Model file for the job. Use its own axes, mm. A direction names the side the tool comes from. Coordinates: 2 decimals unless noted, no trailing zeros. Order: outer loops, then holes, each group sorted by start corner. A loop starts at its lowest first (then second) coordinate and runs counter-clockwise, first axis right, second up. Notation, with made-up numbers: (26, 44.25) -> (60, 44.25) arc R27 cw to (60, 62.25) -> close; hole circle Ø9 at (82.5, 24). An arc over 180 degrees is marked (long way). Return JSON: item names as keys, results as strings. Group by question number.
1) Cut at D-D (z = -16.5). Write the cut outline in (x, y).
2) Flat gauge pins, fed straight in: pin 1 (1 mm diameter, centred on x = 3.5, y = 0.5, fed in from +Z); pin 2 (1 mm diameter, centred on y = 1.5, z = -17, fed in from -X). Where does each tip first touch, or does it go through?
3) Cut at A-A (y = 1.6). Write the cut outline in (x, z) (3 decimals), and give its area (3 significant figures).
4) Pull direction X, two halves, no side cores. Call faces 1 (the flat face through (14.42, 1.01, -18.83)), 2 (the cylindrical face through (-21.145, 1.014, -27.287)), 3 (the flat face through (0, 0, -15)): +X half, -X half, draft (parallel to the pull), parting line (faces both ways), or undercut.
5) Probe line 1 (Z direction, x = -14.5, y = 1.6); line 2 (X direction, y = 0.4, z = -23.5); line 3 (Z direction, x = -14, y = 1.7). List the from-to ranges inside material, lowest first.
6) Which spindle directions (+Z, -Z, +X, -X, +Y, -Y) get a long thin tool onto all of the face, cutting with end or side? Do faces 4 (the cylindrical face through (-19.607, 1.014, -22.597)), 5 (the cylindrical face through (10.805, 1.014, -26.908)), 6 (the flat face through (-14.387, 1.014, -18.877)), 7 (the flat face through (25.863, 1, -26)). Say none if no direction does.
7) Cut at B-B (z = -25.75). Write the cut outline in (x, y), and give its area (3 significant figures).
8) Cut at C-C (x = 0). Write the cut outline in (y, z) (3 decimals).
from build123d import *

# Parameters (mm, degrees)
BOSS_EXTRUDE1_DEPTH = 2
SKETCH5_W           = 68.030538665
SKETCH5_H           = 29.277015507
CUT_EXTRUDE3_DEPTH  = 2


with BuildPart() as part:
    # Sketch3 → Boss-Extrude1 (new body)
    with BuildSketch(Plane(origin=(0, 0, 0), x_dir=(1, 0, 0), z_dir=(0, 1, 0))):
        with BuildLine():
            Line((-13.637639272, 20.383278482), (-15.860247962, 17.20906431))
            ThreePointArc((-15.860247962, 17.20906431), (-13.666207185, 14.707240293), (-12.875283017, 11.475))
            ThreePointArc((-12.875283017, 11.475), (-10.092914311, 8.804356775), (-6.237643745, 8.908278482))
            ThreePointArc((-6.237643745, 8.908278482), (0, 10.875), (6.237643745, 8.908278482))
            ThreePointArc((6.237643745, 8.908278482), (10.092914311, 8.804356775), (12.875283017, 11.475))
            ThreePointArc((12.875283017, 11.475), (13.666207185, 14.707240293), (15.860247962, 17.20906431))
            Line((15.860247962, 17.20906431), (13.637639272, 20.383278482))
            ThreePointArc((13.637639272, 20.383278482), (19.875283017, 22.35), (26.112926762, 20.383278482))
            Line((26.112926762, 20.383278482), (26.112926762, 31.248240565))
            ThreePointArc((26.112926762, 31.248240565), (21.575193898, 27.634543241), (15.870079226, 28.68406431))
            ThreePointArc((15.870079226, 28.68406431), (10.616247764, 27.083629141), (7, 22.95))
            ThreePointArc((7, 22.95), (0, 15.95), (-7, 22.95))
            ThreePointArc((-7, 22.95), (-10.616247764, 27.083629141), (-15.870079226, 28.68406431))
            ThreePointArc((-15.870079226, 28.68406431), (-21.575193898, 27.634543241), (-26.112926762, 31.248240565))
            Line((-26.112926762, 31.248240565), (-26.112926762, 20.383278482))
            ThreePointArc((-26.112926762, 20.383278482), (-19.875283017, 22.35), (-13.637639272, 20.383278482))
        make_face()
    extrude(amount=BOSS_EXTRUDE1_DEPTH)

    # Sketch5 → Cut-Extrude3 (cut)
    with BuildSketch(Plane(origin=(0, 2, 0), x_dir=(1, 0, 0), z_dir=(0, 1, 0))):
        with Locations((1.906858247, 20.166215681)):
            Rectangle(SKETCH5_W, SKETCH5_H)
        with BuildLine():
            Line((25.862926762, 20.851233112), (25.862926762, 30.337137187))
            ThreePointArc((25.862926762, 30.337137187), (21.222970901, 27.301360666), (15.794718469, 28.432380125))
            ThreePointArc((15.794718469, 28.432380125), (10.741632002, 26.866985754), (7.249777379, 22.893184845))
            ThreePointArc((7.249777379, 22.893184845), (0, 15.7), (-7.249777379, 22.893184845))
            ThreePointArc((-7.249777379, 22.893184845), (-10.741632002, 26.866985754), (-15.794718469, 28.432380125))
            ThreePointArc((-15.794718469, 28.432380125), (-21.222970901, 27.301360666), (-25.862926762, 30.337137187))
            Line((-25.862926762, 30.337137187), (-25.862926762, 20.851233112))
            ThreePointArc((-25.862926762, 20.851233112), (-19.513666923, 22.594121314), (-13.291068525, 20.442371104))
            Line((-13.291068525, 20.442371104), (-15.51453889, 17.266926334))
            ThreePointArc((-15.51453889, 17.266926334), (-13.399579679, 14.735025503), (-12.625477511, 11.528104843))
            ThreePointArc((-12.625477511, 11.528104843), (-9.989809939, 9.032549256), (-6.361359115, 9.126814078))
            ThreePointArc((-6.361359115, 9.126814078), (0, 11.125), (6.361359115, 9.126814078))
            ThreePointArc((6.361359115, 9.126814078), (9.989809939, 9.032549256), (12.625477511, 11.528104843))
            ThreePointArc((12.625477511, 11.528104843), (13.399579679, 14.735025503), (15.51453889, 17.266926334))
            Line((15.51453889, 17.266926334), (13.291068525, 20.442371104))
            ThreePointArc((13.291068525, 20.442371104), (19.513666923, 22.594121314), (25.862926762, 20.851233112))
        make_face(mode=Mode.SUBTRACT)
    extrude(amount=-CUT_EXTRUDE3_DEPTH, mode=Mode.SUBTRACT)


solid = part.part
Answers below:
{
 "1": {"outline": "(-14.65, 0) -> (-3.31, 0) -> (-3.31, 2) -> (-14.65, 2) -> close; (3.31, 0) -> (14.65, 0) -> (14.65, 2) -> (3.31, 2) -> close"},
 "2": {"pin 1": "stops at z = -10.38", "pin 2": "stops at x = -15.51"},
 "3": {"outline": "(-25.863, -30.337) arc R7.25 cw to (-15.795, -28.432) arc R9.75 ccw to (-7.25, -22.893) arc R7.25 cw to (7.25, -22.893) arc R9.75 ccw to (15.795, -28.432) arc R7.25 cw to (25.863, -30.337) -> (25.863, -20.851) arc R11.125 cw to (13.291, -20.442) -> (15.515, -17.267) arc R7.25 cw to (12.625, -11.528) arc R4.75 ccw to (6.361, -9.127) arc R11.125 cw to (-6.361, -9.127) arc R4.75 ccw to (-12.625, -11.528) arc R7.25 cw to (-15.515, -17.267) -> (-13.291, -20.442) arc R11.125 cw to (-25.863, -20.851) -> close", "area": "462 mm^2"},
 "4": {"face 1": "+X half", "face 2": "undercut", "face 3": "draft"},
 "5": {"line 1": "z = -28.31 to -21.22, -18.72 to -16.34", "line 2": "x = -25.86 to -7.57, 7.57 to 25.86", "line 3": "z = -28.22 to -20.92, -19.43 to -15.72"},
 "6": {"face 4": "+Y, -Y", "face 5": "-Z, +Y, -Y", "face 6": "-X, +Y, -Y", "face 7": "+Z, -Z, +X, +Y, -Y"},
 "7": {"outline": "(-25.86, 0) -> (-9.33, 0) -> (-9.33, 2) -> (-25.86, 2) -> close; (9.33, 0) -> (25.86, 0) -> (25.86, 2) -> (9.33, 2) -> close", "area": "66.2 mm^2"},
 "8": {"outline": "(0, -15.7) -> (2, -15.7) -> (2, -11.125) -> (0, -11.125) -> close"}
}
